```python
from build123d import *

# Parameters (mm, degrees)
SKETCH081_R             = 1.6
SKETCH081_R_2           = 11.2
PAD028_DEPTH            = 48
POCKET048_DEPTH         = 42
POCKET049_DEPTH         = 42
SKETCH084_W             = 10.029114
SKETCH084_H             = 77.862412
POCKET050_DEPTH         = 48
BODY018_PLACEMENT_ANGLE = 90


with BuildPart() as part:
    # Sketch081 → Pad028 (new body)
    with BuildSketch(Plane.XY):
        Polygon((133.0786530333, 18), (133.0786530333, -18), (151.9182582148, -36.8396051816), (177.784363, -36.8396051816), (177.784363, 36.8396051816), (151.9182582148, 36.8396051816), align=None)
        with Locations((144.0786530333, 0)):
            Circle(SKETCH081_R, mode=Mode.SUBTRACT)
        with Locations((165.9992734624, 21.92)):
            Circle(SKETCH081_R, mode=Mode.SUBTRACT)
        with Locations((165.9992734624, -21.92)):
            Circle(SKETCH081_R, mode=Mode.SUBTRACT)
        with Locations((165.9992734624, 0)):
            Circle(SKETCH081_R_2, mode=Mode.SUBTRACT)
        with Locations((144.0786530333, 18)):
            Circle(SKETCH081_R, mode=Mode.SUBTRACT)
        with Locations((144.0786530333, -18)):
            Circle(SKETCH081_R, mode=Mode.SUBTRACT)
    extrude(amount=-PAD028_DEPTH)

    # Sketch082 (on Face14 of Pad028) → Pocket048 (cut)
    with BuildSketch(Plane(origin=(0, 0, -48), x_dir=(1, 0, 0), z_dir=(0, 0, -1))):
        Polygon((177.784363, 29.5), (164.784363, 29.5), (137.784363, 2.5), (137.784363, -2.5), (164.784363, -29.5), (177.784363, -29.5), align=None)
    extrude(amount=-POCKET048_DEPTH, mode=Mode.SUBTRACT)

    # Sketch083 (on Face4 of Pocket048) → Pocket049 (cut)
    with BuildSketch(Plane.XY):
        Polygon((157.9182582148, 26.18), (131.7382582148, 0), (157.9182582148, -26.18), (157.9182582148, -40), (107.9182582148, -40), (107.9182582148, 40), (157.9182582148, 40), align=None)
    extrude(amount=-POCKET049_DEPTH, mode=Mode.SUBTRACT)

    # Sketch084 (on Face4 of Pocket049) → Pocket050 (cut)
    with BuildSketch(Plane.XY):
        with Locations((178.339218, -0.178093)):
            Rectangle(SKETCH084_W, SKETCH084_H)
    extrude(amount=-POCKET050_DEPTH, mode=Mode.SUBTRACT)


with BuildPart() as part_1:
    # Body018 placement: moved
    add(part.part.moved(Location((0, 54, 58))).rotate(Axis((0, 54, 58), (0, 0, -1)), BODY018_PLACEMENT_ANGLE))


solid = part_1.part
```
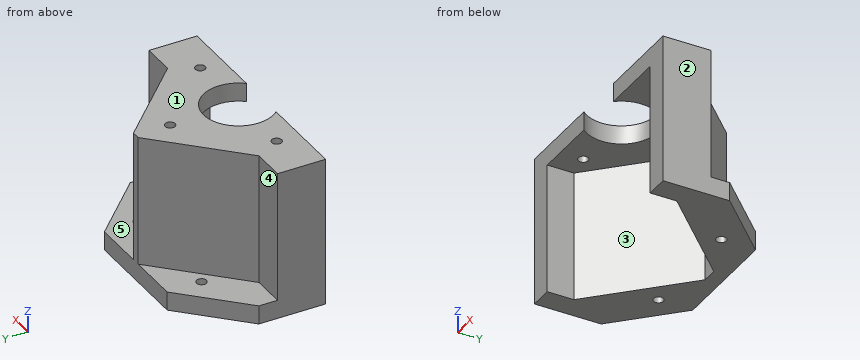
Input: part model. Units: mm. Frame: model coordinates. Face numbers are marked on the shaded views. A direction names the side the tool comes from. Round coordinates to 2 decimals unless told otherwise and drop trailing zeros. Loops run counter-clockwise (first coordinate to the right, second up) from the corner with the lowest first, then second, coordinate; pieces in that order, holes last. Notation, with made-up numbers: (-25, -38) - (-12, -38) arc R9 ccw to (-12, -34) - close; hole circle Ø3 at (-31, 73.25). An arc over 180 degrees is marked (long way). One line per item, written item: value. Start each with the question number.
(1) Section A-A, the plane z = 15. Return loops of the section in (x, y), plus the area to 3 significant figures.
(2) Section B-B, the plane x = 0. Return loops of the section in (y, z).
(3) Contact query for flat-ended pins moving along their axis: P1, Ø5, axis at x = 21.92, y = -112, coming from the -Z side; P2, Ø5, axis at x = 15, z = 27, coming from the -Y side; P3, Ø1.5, axis at x = 7.5, z = 21.5, coming from the +Y side. Output: stop coordinate, or through.
(4) Access query for the marked faces 1, 2, 3, 4 and 5. Directions: +Z, -Z, +X, -X, +Y, -Y. A direction counts if a zero-diameter tool reaches every point of the face in a straight line with its end or side. Return the directions, or none.
(5) Section C-C, the plane y = -109. Return loops of the section in (x, z).
(6) Ray query, line 1 (X direction, y = -116.5, z = 22.5); line 2 (Z direction, x = -20, y = -95); line 3 (Z direction, x = -1, y = -94.5). Return the intervals inside material, ascending. Write a range as [from, to].
(7) Section D-D, the plane z = 51. Return loops of the section in (x, y), plus the area to 3 significant figures.
Results below:
1. outline: (-36.84, -119.32) - (-29.5, -119.32) - (-29.5, -110.78) - (-2.5, -83.78) - (2.5, -83.78) - (29.5, -110.78) - (29.5, -119.32) - (36.84, -119.32) - (36.84, -97.92) - (18, -79.08) - (-18, -79.08) - (-36.84, -97.92) - close; hole circle Ø3.2 at (-18, -90.08); hole circle Ø3.2 at (18, -90.08)
1. area: 1,230 mm^2
2. outline: (-100.8, 52) - (-91.68, 52) - (-91.68, 58) - (-100.8, 58) - close; (-88.48, 52) - (-83.78, 52) - (-83.78, 10) - (-79.08, 10) - (-79.08, 58) - (-88.48, 58) - close
3. P1: z = 52
3. P2: y = -98.78
3. P3: y = -84.49
4. face 1: +Z, +X, -X, +Y, -Y
4. face 2: +Z, -Z, +X, +Y, -Y
4. face 3: -Z, -Y
4. face 4: +Z, -X, +Y
4. face 5: +Z, +X, +Y
5. outline: (-36.84, 10) - (-27.72, 10) - (-27.72, 52) - (-10.79, 52) - (-10.79, 58) - (-36.84, 58) - close; (10.79, 52) - (27.72, 52) - (27.72, 10) - (36.84, 10) - (36.84, 58) - (10.79, 58) - close
6. line 1: [-36.84, -29.5], [29.5, 36.84]
6. line 2: [10, 16]
6. line 3: [52, 58]
7. outline: (-36.84, -119.32) - (-29.5, -119.32) - (-29.5, -110.78) - (-2.5, -83.78) - (2.5, -83.78) - (29.5, -110.78) - (29.5, -119.32) - (36.84, -119.32) - (36.84, -103.92) - (26.18, -103.92) - (1.34, -79.08) - (-1.34, -79.08) - (-26.18, -103.92) - (-36.84, -103.92) - close
7. area: 451 mm^2
